Source: CAD feature listing. Evaluate the final solid. Frame: model axes, mm. A direction names the side the tool comes from. Coordinates: 2 decimals unless noted, no trailing zeros. Loops run counter-clockwise (first coordinate to the right, second up) from the corner with the lowest first, then second, coordinate; pieces in that order, holes last. Notation, with made-up numbers: (49, 56.5) -> (105, 56.5) arc R20 ccw to (105, 72.5) -> close; hole circle Ø8 at (-7, -2.75). An arc over 180 degrees is marked (long way). Answer as CSV lines item,"result".
from build123d import *


with BuildPart() as part:
    # Sketch1 → Revolve1 (revolve)
    with BuildSketch(Plane(origin=(0, 0, 0), x_dir=(0, 0, -1), z_dir=(1, 0, 0))):
        with BuildLine():
            Line((0, 95.25), (12.7, 95.25))
            Line((12.7, 95.25), (12.7, 85.725))
            Line((12.7, 85.725), (9.525, 85.725))
            Line((9.525, 85.725), (9.525, 79.375))
            add(Edge.make_bspline(
                [(9.525, 79.375), (27.523263922, 75.474774462), (31.900002123, 46.864796856), (31.75, 44.45)],
                knots=[0, 0, 0, 0, 1, 1, 1, 1], degree=3))
            Line((31.75, 44.45), (31.75, -95.25))
            Line((31.75, -95.25), (0, -95.25))
            Line((0, -95.25), (0, 95.25))
        make_face()
    revolve(axis=Axis((0, -95.25, 0), (0, 1, 0)))


solid = part.part
(1) Material intervals for L1, parallel to X at y = 37.5, z = -1; L2, parallel to X at y = -78, z = 22; L3, parallel to Y at x = -15.5, z = 18, sorted ascending. Write a range as [from, to].
Computed values:
L1,"[-31.73, 31.73]"
L2,"[-22.89, 22.89]"
L3,"[-95.25, 68.46]"
(2) Cut plane A-A (y = -39). Return the cut outline in (x, z), then the cut area to 3 significant figures.
Computed values:
outline,"circle Ø63.5 at (0, 0)"
area,"3,170 mm^2"
(3) Pin query (flat end, axial travel): pin 1 Ø5 at (y, z) = (16.5, 3.5) entering from -X; pin 2 Ø10 at (x, y) = (-16, -67.5) entering from -Z; pin 3 Ø12 at (y, z) = (63, -23) entering from -X. Return the tip coordinate at first contact, or that it passes through.
Computed values:
pin 1,"x = -31.73"
pin 2,"z = -29.78"
pin 3,"x = -21.6"
(4) Draft query along Y for faces 1 (the flat face through (-9, 85.725, -5)), 2 (the cylindrical face through (5.796, 82.506, 7.559)), 3 (the flat face through (0, -95.25, 0)), 4 (the flat face through (0, 95.25, 0)). Return one class per face: released by +Y, released by -Y, zero draft, split by the parting line, or undercut.
Computed values:
face 1,"undercut"
face 2,"undercut"
face 3,"released by -Y"
face 4,"released by +Y"
(5) Access query for faces 5 (the cylindrical face through (12.4, 90.42, 2.75)), 6 (the cylindrical face through (30.995, -26.378, 6.883)). Directions: +Z, -Z, +X, -X, +Y, -Y. A direction counts if a zero-diameter tool reaches every point of the face in a straight line with its end or side. Return the directions, or none.
Computed values:
face 5,"+Y"
face 6,"+Y, -Y"
